```python
from build123d import *

# Parameters (mm, degrees)
SKETCH2_R          = 1.6
CUT_EXTRUDE1_DEPTH = 15.568802353
CUT_EXTRUDE2_DEPTH = 2


with BuildPart() as part:
    # Sketch1 → Revolve1 (revolve)
    with BuildSketch(Plane(origin=(0, 0, 0), x_dir=(1, 0, 0), z_dir=(0, 1, 0)), mode=Mode.PRIVATE) as revolve1_sk:
        with BuildLine():
            Line((0, 0), (9.5, 0))
            ThreePointArc((9.5, 0), (9.853553391, 0.146446609), (10, 0.5))
            Line((10, 0.5), (10, 1.5))
            ThreePointArc((10, 1.5), (9.853553391, 1.853553391), (9.5, 2))
            Line((9.5, 2), (7, 2))
            Line((7, 2), (6.192982456, 4))
            Line((6.192982456, 4), (4.692982456, 4))
            Line((4.692982456, 4), (4.035087719, 3.5))
            Line((4.035087719, 3.5), (0, 3.5))
            Line((0, 3.5), (0, 0))
        make_face()
    revolve(revolve1_sk.sketch.rotate(Axis((0, 0, -3.5), (0, 0, 1)), 180), axis=Axis((0, 0, -3.5), (0, 0, 1)))

    # Sketch2 → Cut-Extrude1 (cut, through all)
    with BuildSketch(Plane(origin=(0, 0, -3.5), x_dir=(-1, 0, 0), z_dir=(0, 0, -1))):
        Circle(SKETCH2_R)
    extrude(amount=-CUT_EXTRUDE1_DEPTH, mode=Mode.SUBTRACT)

    # Sketch3 → Cut-Extrude2 (cut)
    with BuildSketch(Plane(origin=(0, 0, -3.5), x_dir=(-1, 0, 0), z_dir=(0, 0, -1))):
        Polygon((-1.356166015, -2.807278707), (1.753091669, -2.578113574), (3.109257683, 0.229165133), (1.356166015, 2.807278707), (-1.753091669, 2.578113574), (-3.109257683, -0.229165133), align=None)
    extrude(amount=-CUT_EXTRUDE2_DEPTH, mode=Mode.SUBTRACT)


solid = part.part
```
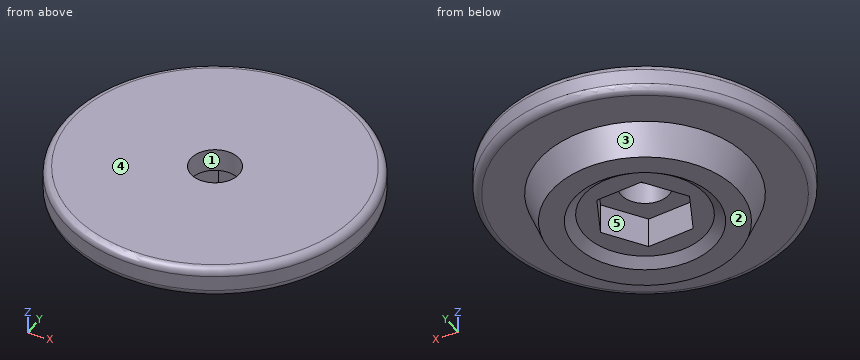
Part model, mm, in its own coordinate system. Face numbers are marked on the shaded views. A direction names the side the tool comes from. Round coordinates to 2 decimals unless told otherwise and drop trailing zeros. Loops run counter-clockwise (first coordinate to the right, second up) from the corner with the lowest first, then second, coordinate; pieces in that order, holes last.
Item 1: Cut at C-C, the plane y = 0. Give the cut face in (x, z), then the cut area to 3 significant figures.
Item 2: Drop flat-ended pins along their axis: P1, Ø1.5, axis at x = 1, y = 3, coming from the -Z side; P2, Ø1.5, axis at x = 2, z = -1.5, coming from the +Y side; P3, Ø1, axis at x = 6, z = -0.5, coming from the -Y side. Give the stop position or say it passes through.
Item 3: 3-axis set-ups, long thin cutter, end or side, ignore diameter. For the marked faces 4 and 5: which of +Z, -Z, +X, -X, +Y, -Y reach the whole face in a straight line?
Item 4: Mould opens along Y. For the marked faces 1, 2 and 3 say: +Y half, -Y half, draft (parallel to the pull), parting line (faces both ways), or undercut.
Item 5: Cut at D-D, the plane z = -0.9. Give the cut face in (x, y).
Item 6: Drill centre lines: line 1 (Y direction, x = 0, z = -0.55); line 2 (Z direction, x = 9, y = 3); line 3 (Y direction, x = 0, z = -0.25). Where is each one in solid material? Low to high.
Item 7: Cut at B-B, the plane x = 0. Give the cut face in (y, z), then the cut area to 3 significant figures.
Item 8: Cut at A-A, the plane z = -2.35. Give the cut face in (x, y).
A:
1. outline: (-10, -1.5) arc R0.5 ccw to (-9.5, -2) - (-7, -2) - (-6.19, -4) - (-4.69, -4) - (-4.04, -3.5) - (-3, -3.5) - (-3, -1.5) - (-1.6, -1.5) - (-1.6, 0) - (-9.5, 0) arc R0.5 ccw to (-10, -0.5) - close; (1.6, -1.5) - (3, -1.5) - (3, -3.5) - (4.04, -3.5) - (4.69, -4) - (6.19, -4) - (7, -2) - (9.5, -2) arc R0.5 ccw to (10, -1.5) - (10, -0.5) arc R0.5 ccw to (9.5, 0) - (1.6, 0) - close
1. area: 45.0 mm2
2. P1: stops at z = -3.5
2. P2: stops at y = 9.92
2. P3: stops at y = -8.35
3. face 4: +Z, +X, -X, +Y, -Y
3. face 5: -Z
4. face 1: undercut
4. face 2: draft
4. face 3: parting line
5. outline: circle Ø20 at (0, 0); hole circle Ø3.2 at (0, 0)
6. line 1: y = -10 to -1.6, 1.6 to 10
6. line 2: z = -2 to 0
6. line 3: y = -9.93 to -1.6, 1.6 to 9.93
7. outline: (-10, -1.5) arc R0.5 ccw to (-9.5, -2) - (-7, -2) - (-6.19, -4) - (-4.69, -4) - (-4.04, -3.5) - (-2.71, -3.5) - (-2.71, -1.5) - (-1.6, -1.5) - (-1.6, 0) - (-9.5, 0) arc R0.5 ccw to (-10, -0.5) - close; (1.6, -1.5) - (2.71, -1.5) - (2.71, -3.5) - (4.04, -3.5) - (4.69, -4) - (6.19, -4) - (7, -2) - (9.5, -2) arc R0.5 ccw to (10, -1.5) - (10, -0.5) arc R0.5 ccw to (9.5, 0) - (1.6, 0) - close
7. area: 46.2 mm2
8. outline: circle Ø13.72 at (0, 0); hole (-3.11, 0.23) - (-1.75, -2.58) - (1.36, -2.81) - (3.11, -0.23) - (1.75, 2.58) - (-1.36, 2.81) - close
